Could you check a few things on this model? Use its own coordinates, in mm. A direction names the side the tool comes from. Round coordinates to 2 decimals unless told otherwise and drop trailing zeros. Loops run counter-clockwise (first coordinate to the right, second up) from the corner with the lowest first, then second, coordinate; pieces in that order, holes last. Notation, with made-up numbers: (18, -36) - (57, -36) arc R31 cw to (57, -2) - close; hole circle Ø10 at (21.5, 54). An arc over 180 degrees is marked (long way). Answer as CSV lines item,"result". Start each with the question number.
1) Please list where these lines run through material, in increasing order: line 1 along Y through (x, z) = (25.5, 0); line 2 along Z through (x, y) = (12.5, -14); line 3 along Z through (x, y) = (44.5, -16.5).
2) Suppose I cut it at C-C, the plane x = 24. Write out the boundary of the cut face in (y, z), then the cut area to 3 significant figures.
3) Suppose I cut it at A-A, the plane z = 0. Count the separate pieces of the cut face and the enclosed holes in it, then the cut area to 3 significant figures.
4) We'd pull the mould along Y, two halves only. Please class faces 1 (the face through (28.272, -24.796, 5.506)), 2 (the face through (24.65, -19.524, 4.336)), 3 (the face through (50, -19, -7)): pulls with the +Y half, pulls with the -Y half, needs draft (parallel to the pull), parting line crosses it, or undercut.
5) Which directions (+Z, -Z, +X, -X, +Y, -Y) give clear straight access to the entire face, cutting with the end or side of a thin tool? Please do faces 4 (the face through (27.5, -22.6, -0.1)), 5 (the face through (0, -8, -19)).
6) I'm going to push flat-ended pins straight in: pin 1 Ø8 at (x, y) = (28, 18) entering from +Z; pin 2 Ø2 at (x, y) = (19.5, 7) entering from +Z; pin 3 Ø4 at (x, z) = (30, -8.5) entering from +Y. Where does each tip first touch, or does it pass through?
7) Suppose I cut it at D-D, the plane x = 30. Write out the boundary of the cut face in (y, z), then the cut area to 3 significant figures.
```python
from build123d import *

# Parameters (mm, degrees)
SKETCH1_R                 = 25.4
SKETCH1_R_2               = 20
BOSS_EXTRUDE1_DEPTH       = 50
SKETCH2_R                 = 30
SKETCH2_R_2               = 21
CUT_EXTRUDE1_DEPTH        = 4
FILLET1_R                 = 4
FILLET2_R                 = 4
M6X1_0_TAPPED_HOLE1_D     = 5
M6X1_0_TAPPED_HOLE1_DEPTH = 13.497848452
M6X1_0_TAPPED_HOLE1_TIP   = 1.502151548


# Some blends are built 0.0001 mm under size
with BuildPart() as part:
    # Sketch1 → Boss-Extrude1 (new body)
    with BuildSketch(Plane(origin=(0, 0, 0), x_dir=(0, 0, -1), z_dir=(1, 0, 0))):
        Circle(SKETCH1_R)
        Circle(SKETCH1_R_2, mode=Mode.SUBTRACT)
    extrude(amount=BOSS_EXTRUDE1_DEPTH)

    # Sketch2 → Cut-Extrude1 (cut)
    with BuildSketch(Plane.ZY):
        Circle(SKETCH2_R)
        Circle(SKETCH2_R_2, mode=Mode.SUBTRACT)
    extrude(amount=-CUT_EXTRUDE1_DEPTH, mode=Mode.SUBTRACT)

    # Fillet1
    fillet1_edges = [part.edges().sort_by_distance(p)[0] for p in [
        (4, 0, -21),
    ]]
    fillet(fillet1_edges, radius=FILLET1_R - 0.0001)  # a hair under: the kernel refuses the full size

    # Fillet2
    # the kernel refuses this fillet: 4 mm, written as the material it takes off along each edge
    with BuildSketch(Plane(origin=(4, 0, 0), x_dir=(0, 0, -1), z_dir=(0, 1, 0))) as fillet2_piece_1:
        with BuildLine():
            CenterArc((21.4, -3.144266851), FILLET2_R, 0, 63.256757147)
            Line((25.4, -3.144266851), (25.8, -3.144266851))
            Line((25.8, -3.144266851), (25.8, 0))
            Line((25.8, 0), (25.4, 0.4))
            ThreePointArc((25.4, 0.4), (24.9999, 0.4), (23.37996975, 0.785074034))
            Line((23.37996975, 0.785074034), (23.1999725, 0.427861226))
        make_face()
    revolve(axis=Axis((4, 0, 0), (-1, 0, 0)), mode=Mode.SUBTRACT)

    # M6x1.0 Tapped Hole1
    with Locations(Plane(origin=(0, -25.4, 0), x_dir=(-1, 0, 0), z_dir=(0, -1, 0))):
        with Locations((-30, 0)):
            Hole(M6X1_0_TAPPED_HOLE1_D / 2, depth=M6X1_0_TAPPED_HOLE1_DEPTH)
            with Locations((0, 0, -(M6X1_0_TAPPED_HOLE1_DEPTH + M6X1_0_TAPPED_HOLE1_TIP / 2))):  # 118° drill point
                Cone(0, M6X1_0_TAPPED_HOLE1_D / 2, M6X1_0_TAPPED_HOLE1_TIP, mode=Mode.SUBTRACT)


solid = part.part
```
Filled sheet:
1,line 1,"-25.4 to -20, 20 to 25.4"
1,line 2,"-21.19 to -14.28, 14.28 to 21.19"
1,line 3,"-19.31 to -11.3, 11.3 to 19.31"
2,outline,"circle Ø50.8 at (0, 0); hole circle Ø40 at (0, 0)"
2,area,"770 mm²"
3,separate pieces,"3"
3,enclosed holes,"0"
3,area,"482 mm²"
4,face 1,"parting line crosses it"
4,face 2,"undercut"
4,face 3,"needs draft"
5,face 4,"-Y"
5,face 5,"+Z, -Z, -X, +Y, -Y"
6,pin 1,"z = 21.19"
6,pin 2,"z = 24.68"
6,pin 3,"y = 24.55"
7,outline,"(-25.28, -2.5) arc R25.4 ccw (long way) to (-25.28, 2.5) - (-19.84, 2.5) arc R20 cw (long way) to (-19.84, -2.5) - close"
7,area,"743 mm²"
